Here's how the part is built. I have some questions about the finished solid (model axes, mm). A direction names the side the tool comes from. Round coordinates to 2 decimals unless told otherwise and drop trailing zeros. Loops run counter-clockwise (first coordinate to the right, second up) from the corner with the lowest first, then second, coordinate; pieces in that order, holes last. Notation, with made-up numbers: M -21,-1 L 23,-1 A15 cw 23,6 Z; hole C 5,39.5 d6. An arc over 180 degrees is marked long. Use a Markdown table: item, result.
```python
from build123d import *

# Parameters (mm, degrees)
SKETCH_1_W          = 140
SKETCH_1_H          = 75
EXTRUDE_1_DEPTH     = 61
SHELL_1_T           = -1.5
SKETCH_3_W          = 130
SKETCH_3_H          = 65
CUT_EXTRUDE_1_DEPTH = 117.308601118
SKETCH_4_W          = 137
SKETCH_4_H          = 2.6
SKETCH_4_H_2        = 3.3
EXTRUDE_2_DEPTH     = 5
SKETCH_5_W          = 2.4
SKETCH_5_H          = 69.4
EXTRUDE_3_DEPTH     = 5
SKETCH_20_W         = 3.5
SKETCH_20_H         = 3.5
EXTRUDE_4_DEPTH     = 6.6
SKETCH_21_R         = 1
EXTRUDE_5_DEPTH     = 5
SKETCH_22_W         = 140
SKETCH_22_H         = 61
SKETCH_22_W_2       = 29.5
SKETCH_22_H_2       = 51.5
CUT_EXTRUDE_4_DEPTH = 100
SKETCH_23_W         = 29.5
SKETCH_23_H         = 51.5
CUT_EXTRUDE_5_DEPTH = 1


with BuildPart() as part:
    # 草图1 → 凸台-拉伸1 (new body)
    with BuildSketch(Plane.XY):
        with Locations((19.248188406, -5.412137681)):
            Rectangle(SKETCH_1_W, SKETCH_1_H)
    extrude(amount=EXTRUDE_1_DEPTH)

    # 抽壳1
    shell_1_openings = [part.faces().sort_by_distance(p)[0] for p in [
        (19.248188406, -5.412137681, 61),
    ]]
    offset(amount=SHELL_1_T, openings=shell_1_openings, kind=Kind.INTERSECTION)

    # 草图3 → 切除-拉伸1 (cut, through all)
    with BuildSketch(Plane(origin=(0, 0, 0), x_dir=(-1, 0, 0), z_dir=(0, 0, -1))):
        with Locations((-19.248188406, -5.412137681)):
            Rectangle(SKETCH_3_W, SKETCH_3_H)
    extrude(amount=-CUT_EXTRUDE_1_DEPTH, mode=Mode.SUBTRACT)

    # 草图4 → 凸台-拉伸2 (add)
    with BuildSketch(Plane.XY.offset(1.5)):
        with Locations((19.248188406, -40.112137681)):
            Rectangle(SKETCH_4_W, SKETCH_4_H)
        with Locations((19.248188406, 28.937862319)):
            Rectangle(SKETCH_4_W, SKETCH_4_H_2)
    extrude(amount=EXTRUDE_2_DEPTH)

    # 草图5 → 凸台-拉伸3 (add)
    with BuildSketch(Plane.XY.offset(1.5)):
        with Locations((-48.051811594, -4.112137681)):
            Rectangle(SKETCH_5_W, SKETCH_5_H)
        with Locations((86.548188406, -4.112137681)):
            Rectangle(SKETCH_5_W, SKETCH_5_H)
    extrude(amount=EXTRUDE_3_DEPTH)

    # 草图20 → 凸台-拉伸4 (add)
    with BuildSketch(Plane(origin=(0, -41.412137681, 0), x_dir=(1, 0, 0), z_dir=(0, 1, 0))):
        with Locations((1.25, -55.75)):
            Rectangle(SKETCH_20_W, SKETCH_20_H)
        with Locations((1.25, -9.75)):
            Rectangle(SKETCH_20_W, SKETCH_20_H)
        with Locations((23.25, -9.75)):
            Rectangle(SKETCH_20_W, SKETCH_20_H)
        with Locations((23.25, -55.75)):
            Rectangle(SKETCH_20_W, SKETCH_20_H)
    extrude(amount=EXTRUDE_4_DEPTH)

    # 草图21 → 凸台-拉伸5 (add)
    with BuildSketch(Plane(origin=(0, -34.812137681, 0), x_dir=(1, 0, 0), z_dir=(0, 1, 0))):
        with Locations(Location((1.25, -55.75, 0), (0, 0, 270))):
            Circle(SKETCH_21_R)
        with Locations(Location((1.25, -9.75, 0), (0, 0, 270))):
            Circle(SKETCH_21_R)
        with Locations(Location((23.25, -9.75, 0), (0, 0, 270))):
            Circle(SKETCH_21_R)
        with Locations(Location((23.25, -55.75, 0), (0, 0, 270))):
            Circle(SKETCH_21_R)
    extrude(amount=EXTRUDE_5_DEPTH)

    # 草图22 → 切除-拉伸4 (cut, symmetric)
    with BuildSketch(Plane(origin=(0, -41.412137681, 0), x_dir=(1, 0, 0), z_dir=(0, 1, 0))):
        with Locations((19.248188406, -30.5)):
            Rectangle(SKETCH_22_W, SKETCH_22_H)
        with Locations((12.25, -32.75)):
            Rectangle(SKETCH_22_W_2, SKETCH_22_H_2, mode=Mode.SUBTRACT)
    extrude(amount=CUT_EXTRUDE_4_DEPTH, both=True, mode=Mode.SUBTRACT)


with BuildPart() as cut_extrude_4_kept_piece:
    # of the separate pieces the step leaves, the one the design keeps (cut_extrude_4_pieces_kept)
    add(part.part.solids().sort_by_distance((27, -42.912137681, 7))[0])

    # 草图23 → 切除-拉伸5 (cut)
    with BuildSketch(Plane.XZ.offset(42.912137681)):
        with Locations((12.25, 32.75)):
            Rectangle(SKETCH_23_W, SKETCH_23_H)
    extrude(amount=-CUT_EXTRUDE_5_DEPTH, mode=Mode.SUBTRACT)


solid = cut_extrude_4_kept_piece.part
```
Q1. Imagine slicing it at A-A, the plane y = -40. Please give me the cut outline in (x, z), then the cut area to 3 significant figures.
Return value:
| item | result |
|---|---|
| outline | M -0.5,8 L 3,8 L 3,11.5 L -0.5,11.5 Z; M -0.5,54 L 3,54 L 3,57.5 L -0.5,57.5 Z; M 21.5,8 L 25,8 L 25,11.5 L 21.5,11.5 Z; M 21.5,54 L 25,54 L 25,57.5 L 21.5,57.5 Z |
| area | 49.0 mm^2 |
Q2. Imagine slicing it at D-D, the plane y = -34.25. Please give me the cut outline in (x, z).
Return value:
| item | result |
|---|---|
| outline | C 1.25,9.75 d2; C 1.25,55.75 d2; C 23.25,9.75 d2; C 23.25,55.75 d2 |
Q3. I need wall thicknesses on line 1 (Z direction, x = 21.75, y = -36.5); line 2 (X direction, y = -35, z = 56.5); line 3 (Y direction, x = 7, z = 24.5). Which ranges of each line are inside material? Lowest first, please. Write a range as from..to.
Return value:
| item | result |
|---|---|
| line 1 | z = 8..11.5, 54..57.5 |
| line 2 | x = -0.5..3, 21.5..25 |
| line 3 | y = -41.91..-41.41 |
Q4. Imagine slicing it at B-B, the plane z = 55.75. Please give me the cut outline in (x, y).
Return value:
| item | result |
|---|---|
| outline | M -2.5,-41.91 L 27,-41.91 L 27,-41.41 L 25,-41.41 L 25,-34.81 L 24.25,-34.81 L 24.25,-29.81 L 22.25,-29.81 L 22.25,-34.81 L 21.5,-34.81 L 21.5,-41.41 L 3,-41.41 L 3,-34.81 L 2.25,-34.81 L 2.25,-29.81 L 0.25,-29.81 L 0.25,-34.81 L -0.5,-34.81 L -0.5,-41.41 L -2.5,-41.41 Z |
Q5. Imagine slicing it at C-C, the plane x = 1.25. Please give me the cut outline in (y, z).
Return value:
| item | result |
|---|---|
| outline | M -41.91,7 L -41.41,7 L -41.41,8 L -34.81,8 L -34.81,8.75 L -29.81,8.75 L -29.81,10.75 L -34.81,10.75 L -34.81,11.5 L -41.41,11.5 L -41.41,54 L -34.81,54 L -34.81,54.75 L -29.81,54.75 L -29.81,56.75 L -34.81,56.75 L -34.81,57.5 L -41.41,57.5 L -41.41,58.5 L -41.91,58.5 Z |
Q6. For faces 5 (the flat face through (1, -38, 57.5)), 6 (the cylindrical face through (22.274, -32.347, 9.533)), 7 (the flat face through (21.5, -38, 10)), 8 (the flat face through (1, -38, 11.5)), which set-ups out of +Z, -Z, +X, -X, +Y, -Y let a thin tool reach every point of the face, with its end or its side?
Return value:
| item | result |
|---|---|
| face 5 | +Z, +X, -X, +Y |
| face 6 | +Y |
| face 7 | +Z, -Z, +Y |
| face 8 | +X, -X, +Y |
Q7. Will these pins go through, and if not, where does the flat tip stop? P1, Ø6, axis at x = 8, y = -39.5, coming from the -Z side; P2, Ø1, axis at x = 22.5, y = -37.5, coming from the +Z side; P3, Ø6, axis at x = 15, z = 21, coming from the +Y side; P4, Ø3, axis at x = 2, y = -35, coming from the -Z side.
Return value:
| item | result |
|---|---|
| P1 | stops at z = 7 |
| P2 | stops at z = 57.5 |
| P3 | stops at y = -41.41 |
| P4 | stops at z = 8 |
Q8. We'd pull the mould along X, two halves only. Please class faces 1 (the flat face through (23, -38, 11.5)), 2 (the flat face through (-0.5, -38, 10)), 3 (the cylindrical face through (0.64, -32.35, 8.96)), 4 (the flat face through (25, -38, 56)): pulls with the +X half, pulls with the -X half, needs draft (parallel to the pull), parting line crosses it, or undercut.
Return value:
| item | result |
|---|---|
| face 1 | needs draft |
| face 2 | pulls with the -X half |
| face 3 | undercut |
| face 4 | pulls with the +X half |
